from build123d import *

# Parameters (mm, degrees)
BOSS_EXTRUDE1_DEPTH = 1.1
SKETCH2_R           = 2.75
BOSS_EXTRUDE2_DEPTH = 2.2
CUT_EXTRUDE1_REACH  = 5.3
SKETCH3_R           = 0.5


with BuildPart() as part:
    # Sketch1 → Boss-Extrude1 (new body)
    with BuildSketch(Plane.XY):
        with BuildLine():
            Line((2.243746866, 1.59), (11.743746866, 1.59))
            ThreePointArc((11.743746866, 1.59), (13.333746866, 0), (11.743746866, -1.59))
            Line((11.743746866, -1.59), (2.243746866, -1.59))
            ThreePointArc((2.243746866, -1.59), (-2.75, 0), (2.243746866, 1.59))
        make_face()
    extrude(amount=BOSS_EXTRUDE1_DEPTH)

    # Sketch2 → Boss-Extrude2 (add)
    with BuildSketch(Plane.XY.offset(1.1)):
        Circle(SKETCH2_R)
    extrude(amount=BOSS_EXTRUDE2_DEPTH)

    # Sketch3 → Cut-Extrude1 (cut, up to next)
    with BuildSketch(Plane(origin=(0, 0, 0), x_dir=(-1, 0, 0), z_dir=(0, 0, -1)), mode=Mode.PRIVATE) as cut_extrude1_sk1:
        with Locations((-11.833746866, 0)):
            Circle(SKETCH3_R)
    cut_extrude1_tool1 = extrude(cut_extrude1_sk1.sketch, amount=-CUT_EXTRUDE1_REACH, mode=Mode.PRIVATE) & part.part
    add(cut_extrude1_tool1.solids().sort_by_distance((11.833747, 0, 0))[0], mode=Mode.SUBTRACT)
    # Sketch3 → Cut-Extrude1 (cut, up to next)
    with BuildSketch(Plane(origin=(0, 0, 0), x_dir=(-1, 0, 0), z_dir=(0, 0, -1)), mode=Mode.PRIVATE) as cut_extrude1_sk2:
        with Locations((-9.458746866, 0)):
            Circle(SKETCH3_R)
    cut_extrude1_tool2 = extrude(cut_extrude1_sk2.sketch, amount=-CUT_EXTRUDE1_REACH, mode=Mode.PRIVATE) & part.part
    add(cut_extrude1_tool2.solids().sort_by_distance((9.458747, 0, 0))[0], mode=Mode.SUBTRACT)
    # Sketch3 → Cut-Extrude1 (cut, up to next)
    with BuildSketch(Plane(origin=(0, 0, 0), x_dir=(-1, 0, 0), z_dir=(0, 0, -1)), mode=Mode.PRIVATE) as cut_extrude1_sk3:
        with Locations((-7.083746866, 0)):
            Circle(SKETCH3_R)
    cut_extrude1_tool3 = extrude(cut_extrude1_sk3.sketch, amount=-CUT_EXTRUDE1_REACH, mode=Mode.PRIVATE) & part.part
    add(cut_extrude1_tool3.solids().sort_by_distance((7.083747, 0, 0))[0], mode=Mode.SUBTRACT)


solid = part.part
Build history of the part. All positions in model axes, mm. A direction names the side the tool comes from. Coordinates: 2 decimals unless noted, no trailing zeros. Order: outer loops, then holes, each group sorted by start corner. A loop starts at its lowest first (then second) coordinate and runs counter-clockwise, first axis right, second up. Notation, with made-up numbers: (2.25, 25) -> (12.25, 25) arc R26 ccw to (12.25, 64) -> close; hole circle Ø8 at (18, -20.75). An arc over 180 degrees is marked (long way). One line per item, written item: value.
(1) Slice it at D-D, the plane y = 1.75. List the corners of the cut face in (x, z), plus the area to 3 significant figures.
Checked values:
outline: (-2.12, 0) -> (2.12, 0) -> (2.12, 3.3) -> (-2.12, 3.3) -> close
area: 14.0 mm2
(2) Mould opens along X. For faces 1 (the flat face through (6.9, 1.59, 0.5)), 2 (the cylindrical face through (9.96, 0.02, 0.54)), 3 (the cylindrical face through (13.333, 0.035, 0.542)) say: pulls with the +X half, pulls with the -X half, needs draft (parallel to the pull), parting line crosses it, or undercut.
Checked values:
face 1: needs draft
face 2: undercut
face 3: pulls with the +X half
(3) Slice it at C-C, the plane z = 2.05. List the corners of the cut face in (x, y).
Checked values:
outline: circle Ø5.5 at (0, 0)
(4) Tool access for faces 4 (the cylindrical face through (11.37, -0.19, 0.54)), 5 (the flat face through (7.1, -1.59, 0.5)): list every direction of +Z, -Z, +X, -X, +Y, -Y with a clear straight run to the whole face (end or side of a thin tool).
Checked values:
face 4: +Z, -Z
face 5: +Z, -Z, +X, -Y
(5) Slice it at A-A, the plane y = 0. List the corners of the cut face in (x, z).
Checked values:
outline: (-2.75, 0) -> (6.58, 0) -> (6.58, 1.1) -> (2.75, 1.1) -> (2.75, 3.3) -> (-2.75, 3.3) -> close; (7.58, 0) -> (8.96, 0) -> (8.96, 1.1) -> (7.58, 1.1) -> close; (9.96, 0) -> (11.33, 0) -> (11.33, 1.1) -> (9.96, 1.1) -> close; (12.33, 0) -> (13.33, 0) -> (13.33, 1.1) -> (12.33, 1.1) -> close
(6) Slice it at B-B, the plane x = 3.75. List the corners of the cut face in (y, z).
Checked values:
outline: (-1.59, 0) -> (1.59, 0) -> (1.59, 1.1) -> (-1.59, 1.1) -> close
(7) Probe line 1 (Z direction, x = 4, y = 0); line 2 (X direction, y = 0.2, z = 0.3); line 3 (Y direction, x = 11.5, z = 0.85). List the from-to ranges inside material, lowest first. Write a range as [from, to].
Checked values:
line 1: [0, 1.1]
line 2: [-2.74, 6.63], [7.54, 9], [9.92, 11.38], [12.29, 13.32]
line 3: [-1.59, -0.37], [0.37, 1.59]
(8) Drop flat-ended pins along their axis: pin 1 Ø1 at (y, z) = (1.5, 2.5) entering from -X; pin 2 Ø1 at (y, z) = (2, 2.5) entering from +X; pin 3 Ø0.6 at (x, z) = (5.5, 1) entering from -Y. Give the stop position or say it passes through.
Checked values:
pin 1: x = -2.56
pin 2: x = 2.3
pin 3: y = -1.59
